from build123d import *

# Parameters (mm, degrees)
SKETCH_1_R      = 28
SKETCH_1_R_2    = 2
SKETCH_1_R_3    = 2.08
SKETCH_1_R_4    = 8.75
SKETCH_1_R_5    = 1.25
EXTRUDE_1_DEPTH = 2


with BuildPart() as part:
    # 草图1 → 凸台-拉伸1 (new body)
    with BuildSketch(Plane.XY):
        Circle(SKETCH_1_R)
        with Locations((0, -15)):
            Circle(SKETCH_1_R_2, mode=Mode.SUBTRACT)
        with Locations((-12.990381057, -7.5)):
            Circle(SKETCH_1_R_2, mode=Mode.SUBTRACT)
        with Locations((-12.990381057, 7.5)):
            Circle(SKETCH_1_R_2, mode=Mode.SUBTRACT)
        with Locations((0, 15)):
            Circle(SKETCH_1_R_2, mode=Mode.SUBTRACT)
        with Locations((12.990381057, 7.5)):
            Circle(SKETCH_1_R_2, mode=Mode.SUBTRACT)
        with Locations((12.990381057, -7.5)):
            Circle(SKETCH_1_R_2, mode=Mode.SUBTRACT)
        with Locations((-13.53, 0)):
            Circle(SKETCH_1_R_3, mode=Mode.SUBTRACT)
        with Locations((6.765, 11.717323713)):
            Circle(SKETCH_1_R_3, mode=Mode.SUBTRACT)
        with Locations((6.765, -11.717323713)):
            Circle(SKETCH_1_R_3, mode=Mode.SUBTRACT)
        Circle(SKETCH_1_R_4, mode=Mode.SUBTRACT)
        with Locations((12.351862398, 21.735489304)):
            Circle(SKETCH_1_R_5, mode=Mode.SUBTRACT)
        with Locations((24.9994171, 0.170718032)):
            Circle(SKETCH_1_R_5, mode=Mode.SUBTRACT)
        with Locations((12.647554702, -21.564771273)):
            Circle(SKETCH_1_R_5, mode=Mode.SUBTRACT)
        with Locations((-12.351862398, -21.735489304)):
            Circle(SKETCH_1_R_5, mode=Mode.SUBTRACT)
        with Locations((-24.9994171, -0.170718032)):
            Circle(SKETCH_1_R_5, mode=Mode.SUBTRACT)
        with Locations((-12.647554702, 21.564771273)):
            Circle(SKETCH_1_R_5, mode=Mode.SUBTRACT)
    extrude(amount=EXTRUDE_1_DEPTH)


solid = part.part
Verification items for the finished model (mm, model axes). Coordinates: 2 decimals unless noted, no trailing zeros. Loops run counter-clockwise (first coordinate to the right, second up) from the corner with the lowest first, then second, coordinate; pieces in that order, holes last. Notation, with made-up numbers: (-34, 51.5) -> (-6, 51.5) arc R33 ccw to (-6, 85.5) -> close; hole circle Ø2 at (-14, -20.5). An arc over 180 degrees is marked (long way). Answer as a JSON object with one key per item and string values. Group by question number.
Item 1: Sectioned sample at A-A on y = 15. Record the boundary of the cut face in (x, z), plus the area to 3 significant figures.
Item 2: Sectioned sample at D-D on y = 7.5. Record the boundary of the cut face in (x, z), plus the area to 3 significant figures.
Item 3: Scan lines: probe 1 along X at (y, z) = (-22, 0.55); probe 2 along X at (y, z) = (-7, 0.1); probe 3 along Y at (x, z) = (-12, 1.75). Record each from-to range of solid material in increasing order.
Item 4: Sectioned sample at C-C on z = 1.5. State how many separate pieces and enclosed holes the cut face has, plus the area to 3 significant figures.
Item 5: Sectioned sample at B-B on x = -6.5. Record the boundary of the cut face in (y, z), plus the area to 3 significant figures.
Item 6: Depth check by flat-ended pin: pin 1 (2 mm diameter, centred on x = 25, y = 0.17, fed in from -Z). Enter the tip coordinate at first touch or a pass-through.
Item 7: Mould release check, pull along Y, two halves, no side actions. Record for faces 1 (the cylindrical face through (25.865, -10.724, 0.986)), 2 (the flat face through (6, 7, 0)), 3 (the cylindrical face through (26.154, -0.308, 0.986)): +Y half, -Y half, draft (parallel to the pull), parting line (faces both ways), or undercut.
Evaluation:
{
 "1": {"outline": "(-23.64, 0) -> (-2, 0) -> (-2, 2) -> (-23.64, 2) -> close; (2, 0) -> (23.64, 0) -> (23.64, 2) -> (2, 2) -> close", "area": "86.6 mm²"},
 "2": {"outline": "(-26.98, 0) -> (-14.99, 0) -> (-14.99, 2) -> (-26.98, 2) -> close; (-10.99, 0) -> (-4.51, 0) -> (-4.51, 2) -> (-10.99, 2) -> close; (4.51, 0) -> (10.99, 0) -> (10.99, 2) -> (4.51, 2) -> close; (14.99, 0) -> (26.98, 0) -> (26.98, 2) -> (14.99, 2) -> close", "area": "73.9 mm²"},
 "3": {"probe 1": "x = -17.32 to -13.57, -11.13 to 11.48, 13.82 to 17.32", "probe 2": "x = -27.11 to -14.93, -11.05 to -5.25, 5.25 to 11.05, 14.93 to 27.11", "probe 3": "y = -25.3 to -22.93, -20.54 to -9.24, -5.76 to -1.41, 1.41 to 5.76, 9.24 to 20.5, 22.63 to 25.3"},
 "4": {"separate pieces": "1", "enclosed holes": "16", "area": "2,080 mm²"},
 "5": {"outline": "(-27.24, 0) -> (-5.86, 0) -> (-5.86, 2) -> (-27.24, 2) -> close; (5.86, 0) -> (27.24, 0) -> (27.24, 2) -> (5.86, 2) -> close", "area": "85.5 mm²"},
 "6": {"pin 1": "passes through"},
 "7": {"face 1": "parting line", "face 2": "draft", "face 3": "undercut"}
}
